Here's how the part is built. I have some questions about the finished solid (model axes, mm). Face numbers are marked on the shaded views. Round coordinates to 2 decimals unless told otherwise and drop trailing zeros. Loops run counter-clockwise (first coordinate to the right, second up) from the corner with the lowest first, then second, coordinate; pieces in that order, holes last. Notation, with made-up numbers: M 67,48 L 81,48 A27 cw 81,64 Z; hole C 45.25,-39 d11. An arc over 180 degrees is marked long. Use a Markdown table: item, result.
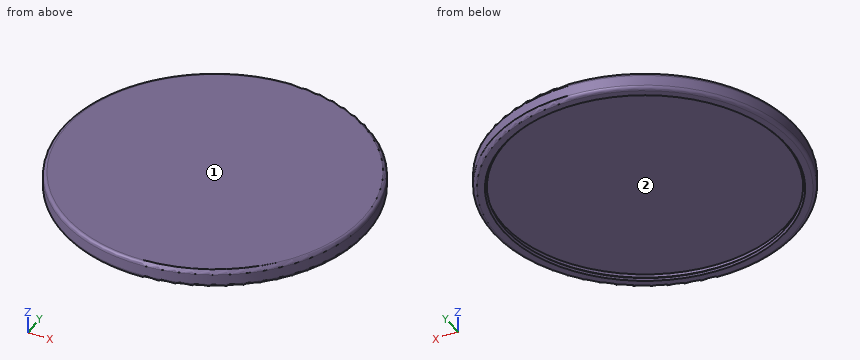
from build123d import *

# Parameters (mm, degrees)
F0_R     = 43.5
F0_R_2   = 40.5
F1_DEPTH = 2
F2_R     = 43.5
F3_DEPTH = 3
F6_R     = 1


with BuildPart() as f1:
    # F0 (on Top) → F1 (new body)
    with BuildSketch(Plane.XY):
        Circle(F0_R)
        Circle(F0_R_2, mode=Mode.SUBTRACT)
    extrude(amount=F1_DEPTH)

    # F2 (on face) → F3 (join)
    with BuildSketch(Plane.XY.offset(2)):
        Circle(F2_R)
    extrude(amount=F3_DEPTH)

    # F4 (on Front) → F5 (revolve)
    with BuildSketch(Plane.XZ):
        Polygon((40, 0.5), (40.5, 0), (40.5, 1), align=None)
    revolve(axis=Axis((0, 0, -3.5082), (0, 0, -1)))

    # F6
    f6_edges = [f1.edges().sort_by_distance(p)[0] for p in [
        (-43.5, 0, 5),
        (-43.5, 0, 0),
    ]]
    fillet(f6_edges, radius=F6_R)


solid = f1.part
1. We'd pull the mould along Y, two halves only. Please class the marked faces 1 and 2: +Y half, -Y half, draft (parallel to the pull), parting line (faces both ways), or undercut.
Answer sheet:
| item | result |
|---|---|
| face 1 | draft |
| face 2 | undercut |
2. I need wall thicknesses on probe 1 along Y at (x, z) = (0, 1.6); probe 2 along Z at (x, y) = (-34, -6.5); probe 3 along X at (y, z) = (26, 1.75). Which ranges of each line are inside material? Lowest first, please. Write a range as from..to.
Answer sheet:
| item | result |
|---|---|
| probe 1 | -43.5..-40.5, 40.5..43.5 |
| probe 2 | 2..5 |
| probe 3 | -34.87..-31.05, 31.05..34.87 |
3. Imagine slicing it at A-A, the plane x = 0. Write out the boundary of the cut face in (y, z), then the cut area to 3 significant figures.
Answer sheet:
| item | result |
|---|---|
| outline | M -43.5,1 A1 ccw -42.5,0 L -40.5,0 L -40,0.5 L -40.5,1 L -40.5,2 L 40.5,2 L 40.5,1 L 40,0.5 L 40.5,0 L 42.5,0 A1 ccw 43.5,1 L 43.5,4 A1 ccw 42.5,5 L -42.5,5 A1 ccw -43.5,4 Z |
| area | 273 mm2 |
4. For pin 1 Ø2 at (x, z) = (-21.5, 4) entering from +Y; pin 2 Ø2 at (x, z) = (10, 4) entering from -Y; pin 3 Ø1.5 at (x, z) = (28.5, 0.5) entering from -Y, each with a flat end and sliding along its axis, tell me the tip position at first contact or that it passes through.
Answer sheet:
| item | result |
|---|---|
| pin 1 | y = 38.37 |
| pin 2 | y = -42.56 |
| pin 3 | y = -33.42 |
